Geometry check sheet. Reference: the model listing, model coordinates, mm. Round coordinates to 2 decimals unless told otherwise and drop trailing zeros. Loops run counter-clockwise (first coordinate to the right, second up) from the corner with the lowest first, then second, coordinate; pieces in that order, holes last. Notation, with made-up numbers: (54, 28.25) -> (86, 28.25) arc R19 cw to (86, 60.25) -> close; hole circle Ø5 at (-7.5, 71). An arc over 180 degrees is marked (long way). Use one line per item in the form item = value.
from build123d import *

# Parameters (mm, degrees)
RESSALTO_EXTRUS_O1_DEPTH                             = 4
FURO_ROSCADO_DE_M21_D                                = 1.6
ESCAREADO_PARA_PARAFUSO_COM_CABE_A_ESCAR_D           = 2.4
ESCAREADO_PARA_PARAFUSO_COM_CABE_A_ESCAR_CSINK_D     = 4.4
ESCAREADO_PARA_PARAFUSO_COM_CABE_A_ESCAR_CSINK_ANGLE = 90
PADR_OCIRCULAR1_COUNT                                = 3


with BuildPart() as part:
    # Esboço1 → Ressalto-extrusão1 (new body)
    with BuildSketch(Plane.XY):
        with BuildLine():
            Line((-5.5, 0), (-5.5, -23))
            Line((-5.5, -23), (5.5, -23))
            Line((5.5, -23), (5.5, 0))
            ThreePointArc((5.5, 0), (0, 5.5), (-5.5, 0))
        make_face()
    extrude(amount=RESSALTO_EXTRUS_O1_DEPTH)

    # Furo roscado de M21 (through all)
    with Locations(Plane(origin=(-4, -20.5, 4), x_dir=(1, 0, 0), z_dir=(0, 0, 1))):
        with Locations((0, 0), (8, 0)):
            Hole(FURO_ROSCADO_DE_M21_D / 2)

    # Escareado para parafuso com cabeça escareada chata de M21 (through all)
    with Locations(Plane(origin=(0, 3, 4), x_dir=(1, 0, 0), z_dir=(0, 0, 1))):
        with Locations((0, 0)):
            escareado_para_parafuso_com_cabe_a_escar = CounterSinkHole(ESCAREADO_PARA_PARAFUSO_COM_CABE_A_ESCAR_D / 2, ESCAREADO_PARA_PARAFUSO_COM_CABE_A_ESCAR_CSINK_D / 2, counter_sink_angle=ESCAREADO_PARA_PARAFUSO_COM_CABE_A_ESCAR_CSINK_ANGLE)

    # PadrãoCircular1: Escareado para parafuso com cabeça escareada chata de M21 ×3 about axis
    padr_ocircular1_axis = Axis((0, 0, 0), (0, 0, 1))
    for i in range(1, PADR_OCIRCULAR1_COUNT):
        add(escareado_para_parafuso_com_cabe_a_escar.rotate(padr_ocircular1_axis, i * 360 / PADR_OCIRCULAR1_COUNT), mode=Mode.SUBTRACT)


solid = part.part
1. Mould release check, pull along Y, two halves, no side actions. Record for faces 1 (the cylindrical face through (0.1, 5.5, 2)), 2 (the cylindrical face through (1.453, -1.14, 1.479)), 3 (the flat face through (0, -9, 0)): released by +Y, released by -Y, zero draft, split by the parting line, or undercut.
Return value:
face_1 = released by +Y
face_2 = undercut
face_3 = zero draft
2. Section check D-D (z = 2.05). Record the boundary of the cut face in (x, y).
Return value:
outline = (-5.5, -23) -> (5.5, -23) -> (5.5, 0) arc R5.5 ccw to (-5.5, 0) -> close; hole circle Ø1.6 at (-4, -20.5); hole circle Ø2.4 at (-2.6, -1.5); hole circle Ø2.4 at (0, 3); hole circle Ø2.4 at (2.6, -1.5); hole circle Ø1.6 at (4, -20.5)
3. Section check A-A (y = -1.5). Record the boundary of the cut face in (x, z).
Return value:
outline = (-5.5, 0) -> (-3.8, 0) -> (-3.8, 3) -> (-4.8, 4) -> (-5.5, 4) -> close; (-1.4, 0) -> (1.4, 0) -> (1.4, 3) -> (0.4, 4) -> (-0.4, 4) -> (-1.4, 3) -> close; (3.8, 0) -> (5.5, 0) -> (5.5, 4) -> (4.8, 4) -> (3.8, 3) -> close
4. Gauge pin test, flat ends, axial feed: pin 1 (3 mm diameter, centred on x = -2.6, y = -1.5, fed in from -Z); pin 2 (1.9 mm diameter, centred on x = 2.6, y = -1.5, fed in from -Z); pin 3 (2 mm diameter, centred on y = 2.5, z = 3, fed in from +X). Record the tip position at first contact, or that the pin passes through.
Return value:
pin_1 = 0
pin_2 = through
pin_3 = 5.29
5. Material ranges on line 1 along Y through (x, z) = (0, 2.45); line 2 along Y through (x, z) = (3.75, 3.85); line 3 along X through (y, z) = (-20, 3.75), recorded low to high.
Return value:
line_1 = -23 to 1.8, 4.2 to 5.5
line_2 = -23 to -21.26, -19.74 to -3.2, 0.2 to 4.02
line_3 = -5.5 to -4.62, -3.38 to 3.38, 4.62 to 5.5
6. Section check B-B (x = 0). Record the boundary of the cut face in (y, z).
Return value:
outline = (-23, 0) -> (1.8, 0) -> (1.8, 3) -> (0.8, 4) -> (-23, 4) -> close; (4.2, 0) -> (5.5, 0) -> (5.5, 4) -> (5.2, 4) -> (4.2, 3) -> close
7. Section check C-C (y = -20.5). Record the boundary of the cut face in (x, z).
Return value:
outline = (-5.5, 0) -> (-4.8, 0) -> (-4.8, 4) -> (-5.5, 4) -> close; (-3.2, 0) -> (3.2, 0) -> (3.2, 4) -> (-3.2, 4) -> close; (4.8, 0) -> (5.5, 0) -> (5.5, 4) -> (4.8, 4) -> close
